Design review of the part built by this model. Coordinates are the model's own, in mm. Coordinates: 2 decimals unless noted, no trailing zeros. Order: outer loops, then holes, each group sorted by start corner. A loop starts at its lowest first (then second) coordinate and runs counter-clockwise, first axis right, second up. Notation, with made-up numbers: M -7.75,74.5 L 38.25,74.5 A30 ccw 38.25,102.5 Z; hole C 15.25,24.25 d1. An arc over 180 degrees is marked long. Answer as a JSON object with one key per item and string values.
from build123d import *

# Parameters (mm, degrees)
ESBO_O1_R                = 1.5
RESSALTO_EXTRUS_O1_DEPTH = 3


with BuildPart() as part:
    # Esboço1 → Ressalto-extrusão1 (new body)
    with BuildSketch(Plane.XY):
        Polygon((22.3, -30), (22.3, -25), (23.675, -25), (23.675, -22.5), (22.3, -22.5), (22.3, -17), (19.3, -17), (19.3, -22.5), (17.925, -22.5), (17.925, -25), (19.3, -25), (19.3, -30), (-3.8, -30), (-3.8, -33), (-11.8, -33), (-11.8, -30), (-11.8, 8.3), (-11.8, 30), (-9.3, 30), (-9.3, 25), (-10.675, 25), (-10.675, 22.5), (-9.3, 22.5), (-9.3, 17), (-6.3, 17), (-6.3, 22.5), (-4.925, 22.5), (-4.925, 25), (-6.3, 25), (-6.3, 30), (16.8, 30), (16.8, 33), (24.8, 33), (24.8, -30), align=None)
        Circle(ESBO_O1_R, mode=Mode.SUBTRACT)
        with Locations((13, 0)):
            Circle(ESBO_O1_R, mode=Mode.SUBTRACT)
    extrude(amount=RESSALTO_EXTRUS_O1_DEPTH)


solid = part.part
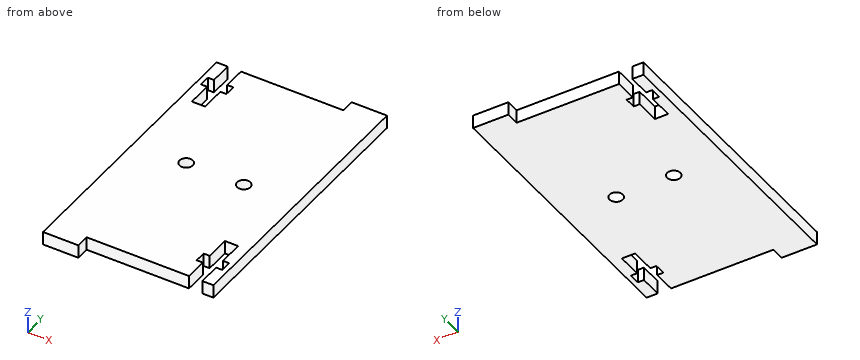
1) Add section A-A (y = 0). State the section outline as (x, z) points, and give its area (3 significant figures).
Taken from the geometry:
{"outline": "M -11.8,0 L -1.5,0 L -1.5,3 L -11.8,3 Z; M 1.5,0 L 11.5,0 L 11.5,3 L 1.5,3 Z; M 14.5,0 L 24.8,0 L 24.8,3 L 14.5,3 Z", "area": "91.8 mm2"}
2) To check wall thickness, follow L1, parallel to X at y = 29.5, z = 1.7; L2, parallel to Y at x = 0, z = 1.2; L3, parallel to Y at x = 7, z = 0.4. State the ranges of each line that lie inside material, in increasing order.
Taken from the geometry:
{"L1": "x = -11.8 to -9.3, -6.3 to 24.8", "L2": "y = -30 to -1.5, 1.5 to 30", "L3": "y = -30 to 30"}
3) Add section D-D (y = 19). State the section outline as (x, z) points.
Taken from the geometry:
{"outline": "M -11.8,0 L -9.3,0 L -9.3,3 L -11.8,3 Z; M -6.3,0 L 24.8,0 L 24.8,3 L -6.3,3 Z"}
4) Insertion check: pin 1 Ø1.5 at (x, z) = (18.5, 2) entering from -Y; pin 2 Ø1.5 at (x, z) = (-5.5, 2) entering from +Y. Each pin has a flat end and moves straight along its axis. Give the tip position at first contact, or say it passes through.
Taken from the geometry:
{"pin 1": "stops at y = -30", "pin 2": "stops at y = 30"}
5) Add section C-C (x = 13). State the section outline as (y, z) points.
Taken from the geometry:
{"outline": "M -30,0 L -1.5,0 L -1.5,3 L -30,3 Z; M 1.5,0 L 30,0 L 30,3 L 1.5,3 Z"}
6) Add section B-B (z = 0.9). Count the separate pieces of the cut face and the enclosed holes in it, and give its area (3 significant figures).
Taken from the geometry:
{"separate pieces": "1", "enclosed holes": "2", "area": "2,140 mm2"}
